```python
from build123d import *

# Parameters (mm, degrees)
SKETCH1_W             = 55.25
SKETCH1_H             = 12.7
BOSS_EXTRUDE1_DEPTH   = 12.7
M5X0_8_TAPPED_HOLE1_D = 4.2
CUT_EXTRUDE1_DEPTH    = 32.060475286
SKETCH5_W             = 18
SKETCH5_H             = 12.7
BOSS_EXTRUDE2_DEPTH   = 1
FILLET1_R             = 1


with BuildPart() as part:
    # Sketch1 → Boss-Extrude1 (new body)
    with BuildSketch(Plane.XY):
        Rectangle(SKETCH1_W, SKETCH1_H)
    extrude(amount=BOSS_EXTRUDE1_DEPTH)

    # M5x0.8 Tapped Hole1 (through all)
    with Locations(Plane(origin=(-20, 6.35, 6.35), x_dir=(0, 0, 1), z_dir=(0, 1, 0))):
        with Locations((0, 0), (0, 40)):
            Hole(M5X0_8_TAPPED_HOLE1_D / 2)

    # Sketch4 → Cut-Extrude1 (cut, through all)
    with BuildSketch(Plane.XY.offset(12.7)):
        with BuildLine():
            ThreePointArc((0, 3.913118961), (-8.75, 0), (0, -3.913118961))
            ThreePointArc((0, -3.913118961), (8.75, 0), (0, 3.913118961))
        make_face()
    extrude(amount=-CUT_EXTRUDE1_DEPTH, mode=Mode.SUBTRACT)

    # Sketch5 → Boss-Extrude2 (add)
    with BuildSketch(Plane(origin=(0, 6.35, 0), x_dir=(1, 0, 0), z_dir=(0, 1, 0))):
        with Locations((0, -6.35)):
            Rectangle(SKETCH5_W, SKETCH5_H)
    boss_extrude2 = extrude(amount=BOSS_EXTRUDE2_DEPTH)

    # Mirror1: Boss-Extrude2 across plane
    add(boss_extrude2.mirror(Plane.ZX))

    # Fillet1
    fillet1_edges = [part.edges().sort_by_distance(p)[0] for p in [
        (9, -7.35, 6.35),
        (-9, -7.35, 6.35),
        (-9, 7.35, 6.35),
        (9, 7.35, 6.35),
    ]]
    fillet(fillet1_edges, radius=FILLET1_R - 0.0001)  # a hair under: the kernel refuses the full size


solid = part.part
```
Geometry: final body of the model. Coordinates: model frame, mm. A direction names the side the tool comes from. Give positions to 0.01 mm unless a question says otherwise; leave off trailing zeros. Loops run counter-clockwise (first coordinate to the right, second up) from the corner with the lowest first, then second, coordinate; pieces in that order, holes last. Notation, with made-up numbers: (77.5, 65) - (89.5, 65) arc R21 cw to (89.5, 77) - close; hole circle Ø6 at (89.25, 87). An arc over 180 degrees is marked (long way). Answer as CSV lines item,"result". Start each with the question number.
(1) Section query D-D (x = 3.5). Output: boundary loops of the cut face in (y, z).
(2) Mould query, pull axis Z, two halves, no side actions, for faces 1 (the face through (0, -7.35, 6)), 2 (the face through (0, 5, 12.7)), 3 (the face through (-17.918, -0.089, 6.623)). Classes: +Z half, -Z half, draft (parallel to the pull), parting line (faces both ways), or undercut.
(3) Section query C-C (z = 5.25). Give the number of separate pieces and of enclosed holes in the cut face, and give its area (3 significant figures).
(4) Section query B-B (x = -20). Output: boundary loops of the cut face in (y, z), and give its area (3 significant figures).
(5) Ray query, line 1 along Y through (x, z) = (-3.5, 7.5); line 2 along X through (y, z) = (3.5, 5.5) (3 decimals); line 3 along X through (y, z) = (-1, 6.35) (3 decimals). Return the intervals inside material, ascending. Write a range as [from, to].
(6) Pin query (flat end, axial travel): P1, Ø4, axis at x = 17, z = 7, coming from the +Y side; P2, Ø1.5, axis at x = -17, z = 2, coming from the -Y side; P3, Ø1, axis at x = -9, z = 5.5, coming from the +Y side; P4, Ø8.5, axis at x = 3.5, y = 0, coming from the -Z side. Return the tip coordinate at first contact, or that it passes through.
(7) Section query A-A (y = 0). Output: boundary loops of the cut face in (x, z) (3 decimals), and give its area (3 significant figures).
(8) Reachability of faces 4 (the face through (18, -6.35, 8)), 5 (the face through (-18, -6.35, 5)), 6 (the face through (18, 6.35, 8)), 7 (the face through (-18, 6.35, 5)) from +Z, -Z, +X, -X, +Y, -Y: full face, straight path, thin tool, end or side. Return the list, or none.
Worked answers:
1,outline,"(-7.35, 0) - (-5.25, 0) - (-5.25, 12.7) - (-7.35, 12.7) - close; (5.25, 0) - (7.35, 0) - (7.35, 12.7) - (5.25, 12.7) - close"
2,face 1,"draft"
2,face 2,"+Z half"
2,face 3,"undercut"
3,separate pieces,"3"
3,enclosed holes,"1"
3,area,"492 mm^2"
4,outline,"(-6.35, 0) - (6.35, 0) - (6.35, 4.25) - (-6.35, 4.25) - close; (-6.35, 8.45) - (6.35, 8.45) - (6.35, 12.7) - (-6.35, 12.7) - close"
4,area,"108 mm^2"
5,line 1,"y = [-7.35, -5.25], [5.25, 7.35]"
5,line 2,"x = [-27.625, -21.92], [-18.08, -7.413], [7.413, 18.08], [21.92, 27.625]"
5,line 3,"x = [-27.625, -22.1], [-17.9, -8.654], [8.654, 17.9], [22.1, 27.625]"
6,P1,"stops at y = 6.35"
6,P2,"stops at y = -6.35"
6,P3,"stops at y = 7.22"
6,P4,"passes through"
7,outline,"(-27.625, 0) - (-8.75, 0) - (-8.75, 12.7) - (-27.625, 12.7) - close; (8.75, 0) - (27.625, 0) - (27.625, 12.7) - (8.75, 12.7) - close; hole circle Ø4.2 at (-20, 6.35); hole circle Ø4.2 at (20, 6.35)"
7,area,"452 mm^2"
8,face 4,"+Z, -Z, +X, -Y"
8,face 5,"+Z, -Z, -X, -Y"
8,face 6,"+Z, -Z, +X, +Y"
8,face 7,"+Z, -Z, -X, +Y"
